from build123d import *

# Parameters (mm, degrees)
SKETCH1_R           = 1.75
SKETCH1_R_2         = 4.318
SKETCH1_W           = 2.032
SKETCH1_H           = 0.508
SKETCH1_R_3         = 3.4
BOSS_EXTRUDE1_DEPTH = 9.525
FILLET1_R           = 6.35
CHAMFER1_SIZE       = 8.89
FILLET2_R           = 2.54


with BuildPart() as part:
    # Sketch1 → Boss-Extrude1 (new body)
    with BuildSketch(Plane(origin=(0, 0, 0), x_dir=(1, 0, 0), z_dir=(0, 1, 0))):
        Polygon((-156.2525, 25.4), (-156.2525, -25.4), (-118.1525, -25.4), (-99.913840717, -63.5), (99.913840717, -63.5), (118.1525, -25.4), (156.2525, -25.4), (156.2525, 25.4), align=None)
        with Locations(Location((-72.438538283, -48.905859703, 0), (0, 0, 90))):
            Circle(SKETCH1_R, mode=Mode.SUBTRACT)
        with Locations(Location((-28.750538283, -45.984859703, 0), (0, 0, 90))):
            Circle(SKETCH1_R, mode=Mode.SUBTRACT)
        with Locations(Location((-150.5375, -12.446, 0), (0, 0, 90))):
            Circle(SKETCH1_R_2, mode=Mode.SUBTRACT)
        with Locations(Location((-28.750538283, -13.980859703, 0), (0, 0, 90))):
            Circle(SKETCH1_R, mode=Mode.SUBTRACT)
        with Locations(Location((93.949510286, 4.876851367, 0), (0, 0, 90))):
            Circle(SKETCH1_R, mode=Mode.SUBTRACT)
        with Locations(Location((0.949510286, 4.876851367, 0), (0, 0, 90))):
            Circle(SKETCH1_R, mode=Mode.SUBTRACT)
        with Locations(Location((0.949510286, -50.123148633, 0), (0, 0, 90))):
            Circle(SKETCH1_R, mode=Mode.SUBTRACT)
        with Locations(Location((93.949510286, -50.123148633, 0), (0, 0, 90))):
            Circle(SKETCH1_R, mode=Mode.SUBTRACT)
        with Locations(Location((150.5375, -12.446, 0), (0, 0, 90))):
            Circle(SKETCH1_R_2, mode=Mode.SUBTRACT)
        with Locations(Location((-150.5375, 12.446, 0), (0, 0, 90))):
            Circle(SKETCH1_R_2, mode=Mode.SUBTRACT)
        with Locations((-50.250952403, 6.442)):
            Rectangle(SKETCH1_W, SKETCH1_H, mode=Mode.SUBTRACT)
        with Locations(Location((-50.250952403, 12.446, 0), (0, 0, 90))):
            Circle(SKETCH1_R_3, mode=Mode.SUBTRACT)
        with Locations(Location((150.5375, 12.446, 0), (0, 0, 90))):
            Circle(SKETCH1_R_2, mode=Mode.SUBTRACT)
    extrude(amount=BOSS_EXTRUDE1_DEPTH)

    # Fillet1
    fillet1_edges = [part.edges().sort_by_distance(p)[0] for p in [
        (118.1525, 4.7625, 25.4),
        (99.913840717, 4.7625, 63.5),
        (-99.913840717, 4.7625, 63.5),
        (-118.1525, 4.7625, 25.4),
    ]]
    fillet(fillet1_edges, radius=FILLET1_R)

    # Chamfer1
    chamfer1_edges = [part.edges().sort_by_distance(p)[0] for p in [
        (156.2525, 4.7625, -25.4),
        (156.2525, 4.7625, 25.4),
        (-156.2525, 4.7625, 25.4),
        (-156.2525, 4.7625, -25.4),
    ]]
    chamfer(chamfer1_edges, length=CHAMFER1_SIZE)

    # Fillet2
    fillet2_edges = [part.edges().sort_by_distance(p)[0] for p in [
        (-156.2525, 4.7625, 16.51),
        (-156.2525, 4.7625, -16.51),
        (147.3625, 4.7625, -25.4),
        (-147.3625, 4.7625, -25.4),
        (-147.3625, 4.7625, 25.4),
        (156.2525, 4.7625, 16.51),
        (156.2525, 4.7625, -16.51),
        (147.3625, 4.7625, 25.4),
    ]]
    fillet(fillet2_edges, radius=FILLET2_R)


solid = part.part
Design review of the part built by this model. Coordinates are the model's own, in mm. A direction names the side the tool comes from. Give positions to 0.01 mm unless a question says otherwise; leave off trailing zeros. Write each loop counter-clockwise with the first axis right and the second up, starting at its lowest first coordinate (ties: lowest second). Pieces come first, ordered by that corner, then holes. Notation, with made-up numbers: M 42,59 L 70,59 A23 cw 70,87 Z; hole C -12,-35.75 d3. An arc over 180 degrees is marked long. Return JSON: item names as keys, results as strings. Group by question number.
Item 1: Take a section at C-C (y = 5.5). Count the separate pieces of the cut face and the enclosed holes in it, plus the area to 3 significant figures.
Item 2: Wall thickness on line 1 along X through (y, z) = (7.5, -12.5); line 2 along X through (y, z) = (5.75, -4.5); line 3 along X through (y, z) = (6.75, 14): over which ranges is each line inside the solid? List them lowest first.
Item 3: The part is to be moulded in two halves that separate along Z. For faces 1 (the flat face through (151.756, 4.696, 21.007)), 2 (the cylindrical face through (154.368, 4.696, -14.438)), 3 (the flat face through (-156.252, 5, 0)), 4 (the cylindrical face through (-154.178, 4.696, 10.125)), say which applies: pulls with the +Z half, pulls with the -Z half, needs draft (parallel to the pull), parting line crosses it, or undercut.
Item 4: Clearance check with flat-ended pins moving along their axes: pin 1 Ø12 at (x, z) = (5.5, 12.5) entering from -Y; pin 2 Ø3 at (x, y) = (128.5, 3.5) entering from +Z. State where each tip first meets the part, or that it passes through.
Item 5: Take a section at B-B (z = 54.5). Give the boundary of the cut face in (x, y) (3 decimals), plus the area to 3 significant figures.
Item 6: Tool access review of faces 5 (the flat face through (-134, 5, 25.4)), 6 (the flat face through (-2, 9.525, 18)), 7 (the flat face through (134, 5, 25.4)): name each direction out of +Z, -Z, +X, -X, +Y, -Y from which nothing blocks a thin tool from reaching the whole face with its end or side.
Item 7: Take a section at A-A (x = -105.5). Give the boundary of the cut face in (y, z) (3 decimals).
Return value:
{
 "1": {"separate pieces": "1", "enclosed holes": "13", "area": "23,700 mm2"},
 "2": {"line 1": "x = -156.25 to -154.86, -146.22 to -53.65, -46.85 to 146.22, 154.86 to 156.25", "line 2": "x = -156.25 to -0.76, 2.66 to 92.24, 95.66 to 156.25", "line 3": "x = -156.25 to -154.57, -146.51 to -30.5, -27 to 146.51, 154.57 to 156.25"},
 "3": {"face 1": "pulls with the +Z half", "face 2": "undercut", "face 3": "needs draft", "face 4": "undercut"},
 "4": {"pin 1": "stops at y = 0", "pin 2": "stops at z = 25.4"},
 "5": {"outline": "M -104.222,0 L 104.222,0 L 104.222,9.525 L -104.222,9.525 Z", "area": "1,990 mm2"},
 "6": {"face 5": "+Z, -X, +Y, -Y", "face 6": "+Z, -Z, +X, -X, +Y", "face 7": "+Z, +X, +Y, -Y"},
 "7": {"outline": "M 0,-25.4 L 9.525,-25.4 L 9.525,51.831 L 0,51.831 Z"}
}
